For this review, take the finished solid that the model builds, in its own axes (mm). A direction names the side the tool comes from. Give positions to 0.01 mm unless a question says otherwise; leave off trailing zeros. Write each loop counter-clockwise with the first axis right and the second up, starting at its lowest first coordinate (ties: lowest second). Pieces come first, ordered by that corner, then holes. Notation, with made-up numbers: M 14,-26 L 64,-26 A21 ccw 64,-10 Z; hole C 66,18.5 d8. An arc over 180 degrees is marked long. Use one line per item in the form item = value. Start each with the question number.
Q1. Tool access review of faces 1 (the flat face through (26, 53.2, 1)), 2 (the cylindrical face through (1.23, 38.25, -0.49)), 3 (the flat face through (52, 45, -5)), 4 (the flat face through (25, 35.2, 1)): name each direction out of +Z, -Z, +X, -X, +Y, -Y from which nothing blocks a thin tool from reaching the whole face with its end or side.
Q2. Consider section C-C on x = 46. Write out the cut boundary in (y, z), and give its area (3 significant figures).
Q3. Mouldability with a two-part tool opening along X and no side actions: class faces 5 (the flat face through (27, 44, 3)), 6 (the flat face through (53.451, 44.7, -4.6)), 7 (the flat face through (21, 44, 0)) as released by +X, released by -X, zero draft, split by the parting line, or undercut.
Q4. Consider section D-D on y = 24. Write out the cut boundary in (x, z), and give its area (3 significant figures).
Q5. Clearance check with flat-ended pins moving along their axes: pin 1 Ø8 at (x, z) = (21.5, -1.5) entering from +Y; pin 2 Ø1.6 at (x, y) = (52, 39.5) entering from -Z; pin 3 Ø10 at (y, z) = (53, -7.5) entering from -X. State where each tip first meets the part, or that it passes through.
Q6. Consider section B-B on y = 52. Write out the cut boundary in (x, z), and give its area (3 significant figures).
Q7. For probe 1 along X at (y, z) = (44, 2); probe 2 along X at (y, z) = (21, 1.5); probe 3 along Y at (x, z) = (23, 0.25), list the stretches that pass through material, from the lowest coordinate up. Write a range as [from, to].
Autodesk Inventor part; units mm, degrees
ref_plane "YZ Plane" through (0, 0, 0) normal (1, 0, 0) x (0, 1, 0)
ref_plane "XZ Plane" through (0, 0, 0) normal (0, 1, 0) x (-1, 0, 0)
ref_plane "XY Plane" through (0, 0, 0) normal (0, 0, 1) x (1, 0, 0)
sketch "Sketch1" plane through (0, 0, 0) normal (0, 0, 1) x (1, 0, 0)
  line L0 (-8.5494, 35.2005) -> (51.4506, 35.2005)
  line L1 (51.4506, 35.2005) -> (51.4506, 53.2005)
  line L2 (51.4506, 53.2005) -> (-8.5494, 53.2005)
  line L3 (-8.5494, 53.2005) -> (-8.5494, 35.2005)
  point P0 (0, 0)
  dimension "d0" = 18
  dimension "d1" = 60
extrude "Extrusion1" add sketch "Sketch1" along normal blind 3
sketch "Sketch2" plane through (0, 0, 0) normal (0, 0, -1) x (-1, 0, 0)
  circle A0 centre (-0.4506, 44.2005) radius 4.5
  line L0 (-0.4506, 44.2005) -> (8.5494, 44.2005) construction
  line L1 (8.5494, 53.2005) -> (8.5494, 35.2005)
  line L2 (-0.4506, 44.2005) -> (-0.4506, 35.2005) construction
  line L3 (8.5494, 35.2005) -> (-51.4506, 35.2005)
  line L4 (-0.4506, 44.2005) -> (-0.4506, 53.2005) construction
  line L5 (-51.4506, 53.2005) -> (8.5494, 53.2005)
  point P0 (0, 0)
  dimension "d4" = 9
extrude "Extrusion2" add sketch "Sketch2" along normal blind 5
sketch "Sketch4" plane through (0.4506, 44.2005, -5) normal (0, 0, -1) x (-1, 0, 0)
  circle A0 centre (0, 0) radius 4.5
  circle A1 centre (0, 0) radius 4
  line L0 (4, -3.1231) -> (4, 2.6998) construction
  point P0 (0.4506, -44.2005)
revolve "Revolution1" [suppressed]
sketch "Sketch5" plane through (0.2094, 44.2005, -3.3681) normal (-0.342, 0, -0.9397) x (-0.9397, 0, 0.342)
  ellipse E0 centre (0, 0) end of major axis (0, -4) minor radius 4
  point P0 (1.3487, -44.2005)
extrude "Extrusion3" [suppressed]
fillet "Fillet1" radius 9 2 edges at (-8.5494, 35.2005, 1.5) (-8.5494, 53.2005, 1.5)
sketch "Sketch6" plane through (51.4506, 35.2005, 0) normal (1, 0, 0) x (0, 0, -1)
  line L0 (-3, 44) -> (17, 44)
  line L1 (17, -26) -> (-3, -26)
  line L2 (-3, -26) -> (-3, 44)
  line L3 (-3, 0) -> (-3, 18)
  line L4 (0, 0) -> (-3, 0)
  line L5 (0, 0) -> (-3, -26) construction
  line L6 (0, 18) -> (-3, 18)
  line L7 (0, 18) -> (-3, 44) construction
  line L8 (17, 44) -> (17, 36)
  line L9 (17, 36) -> (5, 36)
  line L10 (5, 36) -> (5, -18)
  line L11 (5, -18) -> (17, -18)
  line L12 (17, -18) -> (17, -26)
  point P0 (0, -35.2005)
  dimension "d11" = 70
  dimension "d12" = 0
  dimension "d15" = 20
  dimension "d16" = 8
  dimension "d17" = 8
  dimension "d18" = 8
  dimension "d19" = 20
extrude "Extrusion4" add sketch "Sketch6" along normal blind 2
chamfer "Chamfer1" distance 6 angle 45 2 edges at (52.4506, 79.2005, 3) (52.4506, 9.2005, 3)
chamfer "Chamfer2" distance 2 angle 45 2 edges at (52.4506, 17.2005, -5) (52.4506, 71.2005, -5)
fillet "Fillet3" radius 1 13 edges at (52.4506, 17.2005, -17) (52.4506, 9.2005, -17) (52.4506, 79.2005, -17) (52.4506, 71.2005, -17) (52.4506, 71.2005, -7) (52.4506, 69.2005, -5) (52.4506, 19.2005, -5) (52.4506, 17.2005, -7) (52.4506, 79.2005, -3) (52.4506, 9.2005, -3) (51.4506, 53.2005, 1.5) (51.4506, 44.2005, 0) (51.4506, 35.2005, 1.5)
fillet "Fillet4" radius 1 1 edges at (4.9506, 44.2005, -5)
sketch "Sketch7" plane through (0, 0, 0) normal (0, 0, -1) x (-1, 0, 0)
  circle A0 centre (-0.4506, 44.2005) radius 4.5
  circle A1 centre (-0.4506, 44.2005) radius 6
  point P0 (0, 0)
  dimension "d29" = 12
extrude "Extrusion5" add sketch "Sketch7" along normal blind 1 contours A0 | A1
equation "\"d17\" = d16"
equation "\"d18\" = d16"
equation "\"d19\" = d15"
properties part number "Holder"
Working result:
q1.face_1 = +Z, -Z, -X, +Y
q1.face_2 = -Z
q1.face_3 = -Z, +X, -X
q1.face_4 = +Z, -Z, -X, -Y
q2.outline = M 35.2,0 L 53.2,0 L 53.2,3 L 35.2,3 Z
q2.area = 54.0 mm²
q3.face_5 = zero draft
q3.face_6 = released by +X
q3.face_7 = undercut
q4.outline = M 51.45,-5 L 53.45,-5 L 53.45,3 L 51.45,3 Z
q4.area = 16.0 mm²
q5.pin_1 = 53.2
q5.pin_2 = -5
q5.pin_3 = 51.45
q6.outline = M -4.04,0 L 50.45,0 A1 cw 51.45,-1 L 51.45,-5 L 53.45,-5 L 53.45,3 L -4.04,3 Z
q6.area = 183 mm²
q7.probe_1 = [-8.55, 53.45]
q7.probe_2 = [51.45, 53.45]
q7.probe_3 = [35.2, 53.2]
